Work out the finished part from the listing and answer in its coordinate system (mm). Face numbers are marked on the shaded views. A direction names the side the tool comes from. Give positions to 0.01 mm unless a question says otherwise; leave off trailing zeros. Write each loop counter-clockwise with the first axis right and the second up, starting at its lowest first coordinate (ties: lowest second). Pieces come first, ordered by that corner, then holes. Notation, with made-up numbers: (-32.5, 70.25) - (-2.5, 70.25) arc R31 ccw to (-2.5, 98.25) - close; hole circle Ø11 at (-32.5, -39). An arc over 180 degrees is marked (long way). Write each question's results on one line, items separated by ' | '. Start each with the question number.
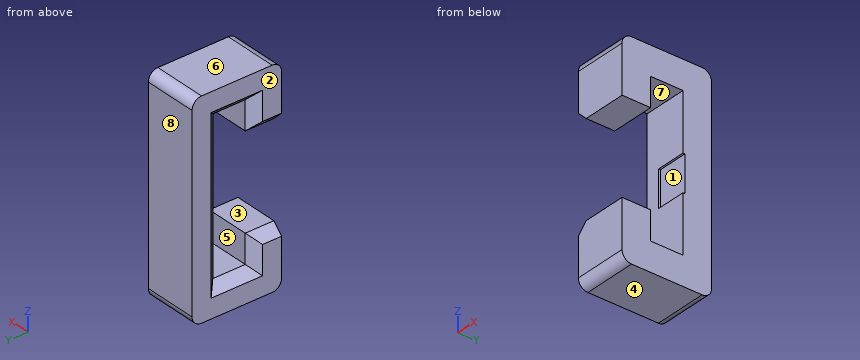
from build123d import *

# Parameters (mm, degrees)
BOSS_EXTRUDE_CLIP_DEPTH       = 2.8
BOSS_EXTRUDE_START            = -2.8
CLIP_OUTLINE_3_W              = 1.9
CLIP_OUTLINE_3_H              = 0.1
BOSS_EXTRUDE_CLIP_NOTCH_DEPTH = 1.240192379
CHAMFER_CLIP_SIZE             = 0.5


with BuildPart() as part:
    # Clip outline → Boss-Extrude clip (new body)
    with BuildSketch(Plane(origin=(0, 0, 0), x_dir=(0, 0, -1), z_dir=(1, 0, 0))):
        with BuildLine():
            Line((-4.95, 2.2), (-2.45, 2.2))
            Line((-2.45, 2.2), (-2.45, 3.7))
            Line((-2.45, 3.7), (-3.95, 3.7))
            Line((-3.95, 3.7), (-3.95, 5.4))
            Line((-3.95, 5.4), (-0.95, 5.4))
            Line((-0.95, 5.4), (-0.95, 5.5))
            Line((-0.95, 5.5), (0.95, 5.5))
            Line((0.95, 5.5), (0.95, 5.4))
            Line((0.95, 5.4), (3.95, 5.4))
            Line((3.95, 5.4), (3.95, 3.7))
            Line((3.95, 3.7), (2.45, 3.7))
            Line((2.45, 3.7), (2.45, 2.2))
            Line((2.45, 2.2), (4.95, 2.2))
            ThreePointArc((4.95, 2.2), (5.303553391, 2.346446609), (5.45, 2.7))
            Line((5.45, 2.7), (5.45, 6.4))
            ThreePointArc((5.45, 6.4), (5.303553391, 6.753553391), (4.95, 6.9))
            Line((4.95, 6.9), (-4.95, 6.9))
            ThreePointArc((-4.95, 6.9), (-5.303553391, 6.753553391), (-5.45, 6.4))
            Line((-5.45, 6.4), (-5.45, 2.7))
            ThreePointArc((-5.45, 2.7), (-5.303553391, 2.346446609), (-4.95, 2.2))
        make_face()
    extrude(amount=-BOSS_EXTRUDE_CLIP_DEPTH)

    # Clip outline<3> → Boss-Extrude clip notch (add)
    with BuildSketch(Plane(origin=(0, 0, 0), x_dir=(0, 0, -1), z_dir=(1, 0, 0)).offset(BOSS_EXTRUDE_START)):
        with Locations((0, 5.45)):
            Rectangle(CLIP_OUTLINE_3_W, CLIP_OUTLINE_3_H)
    extrude(amount=BOSS_EXTRUDE_CLIP_NOTCH_DEPTH)

    # Chamfer clip
    chamfer_clip_edges = [part.edges().sort_by_distance(p)[0] for p in [
        (-2.8, 2.95, 2.45),
        (-2.8, 3.7, 3.2),
        (-2.8, 4.55, 3.95),
        (-2.8, 5.4, 0),
        (-2.8, 4.55, -3.95),
        (-2.8, 3.7, -3.2),
        (-2.8, 2.95, -2.45),
    ]]
    chamfer(chamfer_clip_edges, length=CHAMFER_CLIP_SIZE)


solid = part.part
Q1. A cutting plane is placed at A-A, the plane y = 3.5. Write down the section's boundary in (x, z).
Q2. A cutting plane is placed at B-B, the plane z = 3.5. Write down the section's boundary in (x, y), and give its area (3 significant figures).
Q3. A tool of negligible diameter and unlimited length cuts with its end or side. For the marked faces 1, 2, 3, 4 and 5, from which of +Z, -Z, +X, -X, +Y, -Y can it reach the whole face along a straight path? Write none if from no direction.
Q4. The mould has two halves that part along Y. Classify the marked faces 6, 7 and 8: pulls with the +Y half, pulls with the -Y half, needs draft (parallel to the pull), parting line crosses it, or undercut.
Q5. A cutting plane is placed at C-C, the plane x = -1.05. Write down the section's boundary in (y, z), and give its area (3 significant figures).
Q6. Consider L1, parallel to Y at x = -2.2, z = -3.25; L2, parallel to Z at x = -2, y = 3.95; L3, parallel to Y at x = -0.9, z = -2.25. Determine where each line is inside the solid, lowest interval first.
Q7. A cutting plane is placed at D-D, the plane z = -0.5. Write down the section's boundary in (x, y).
Q8. Given pin 1 (0.5 mm diameter, centred on x = -0.5, z = -0.5, fed in from -Y), flat-ended and moving along its own axis, determine where the tip first touches the part or whether it passes through.
Result:
1) outline: (-2.8, -5.45) - (0, -5.45) - (0, -2.45) - (-2.3, -2.45) - (-2.5, -2.65) - (-2.5, -4.15) - (-2.8, -4.45) - close; (-2.8, 4.45) - (-2.5, 4.15) - (-2.5, 2.65) - (-2.3, 2.45) - (0, 2.45) - (0, 5.45) - (-2.8, 5.45) - close
2) outline: (-2.8, 2.2) - (0, 2.2) - (0, 3.7) - (-2.3, 3.7) - (-2.8, 3.2) - close; (-2.8, 5.9) - (-2.3, 5.4) - (0, 5.4) - (0, 6.9) - (-2.8, 6.9) - close | area: 8.15 mm2
3) face 1: +X, -Y | face 2: +Z, -Z, -X, +Y, -Y | face 3: +X, -X, -Y | face 4: -Z, +X, -X, +Y, -Y | face 5: +X, -X
4) face 6: needs draft | face 7: undercut | face 8: pulls with the +Y half
5) outline: (2.2, -4.95) arc R0.5 ccw to (2.7, -5.45) - (6.4, -5.45) arc R0.5 ccw to (6.9, -4.95) - (6.9, 4.95) arc R0.5 ccw to (6.4, 5.45) - (2.7, 5.45) arc R0.5 ccw to (2.2, 4.95) - (2.2, 2.45) - (3.7, 2.45) - (3.7, 3.95) - (5.4, 3.95) - (5.4, 0.95) - (5.5, 0.95) - (5.5, -0.95) - (5.4, -0.95) - (5.4, -3.95) - (3.7, -3.95) - (3.7, -2.45) - (2.2, -2.45) - close | area: 30.0 mm2
6) L1: y = 2.2 to 3.7, 5.4 to 6.9 | L2: z = -5.45 to -3.95, 3.95 to 5.45 | L3: y = 5.4 to 6.9
7) outline: (-2.8, 5.9) - (-2.3, 5.4) - (-1.56, 5.4) - (-1.56, 5.5) - (0, 5.5) - (0, 6.9) - (-2.8, 6.9) - close
8) pin 1: stops at y = 5.5
